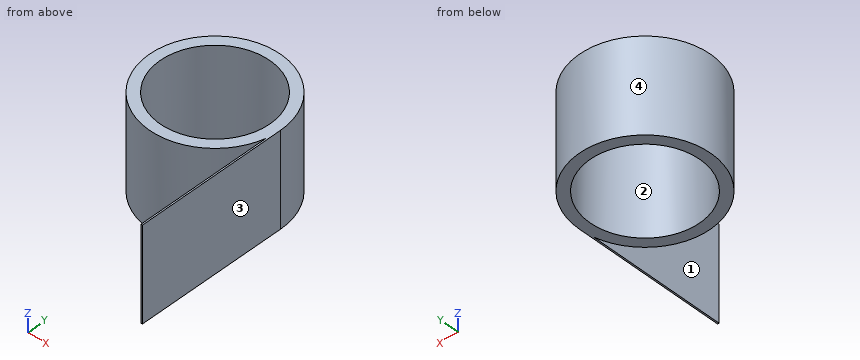
```python
from build123d import *

# Parameters (mm, degrees)
SKETCH1_R           = 11.0871
SKETCH1_R_2         = 9.271
BOSS_EXTRUDE1_DEPTH = 15.875
BOSS_EXTRUDE2_START = -15.875
BOSS_EXTRUDE2_DEPTH = 15.875


with BuildPart() as part:
    # Sketch1 → Boss-Extrude1 (new body)
    with BuildSketch(Plane.XY):
        Circle(SKETCH1_R)
        Circle(SKETCH1_R_2, mode=Mode.SUBTRACT)
    extrude(amount=BOSS_EXTRUDE1_DEPTH)

    # Sketch2 → Boss-Extrude2 (add)
    with BuildSketch(Plane.XY.offset(15.875).offset(BOSS_EXTRUDE2_START)):
        with BuildLine():
            Line((11.0871, 0), (11.0871, -25.4))
            Line((11.0871, -25.4), (10.8331, -25.4))
            Line((10.8331, -25.4), (10.8331, -2.35960395))
            ThreePointArc((10.8331, -2.35960395), (11.023417107, -1.186617756), (11.0871, 0))
        make_face()
    extrude(amount=BOSS_EXTRUDE2_DEPTH)


solid = part.part
```
The model under review builds one solid part; all positions refer to its coordinate system, in mm. Face numbers are marked on the shaded views. A direction names the side the tool comes from. Round coordinates to 2 decimals unless told otherwise and drop trailing zeros. Loops run counter-clockwise (first coordinate to the right, second up) from the corner with the lowest first, then second, coordinate; pieces in that order, holes last. Notation, with made-up numbers: M 80.25,-31.5 L 97.25,-31.5 A15 cw 97.25,-5.5 Z; hole C 58.25,87 d6. An arc over 180 degrees is marked long. Write item = value, one per line.
Item 1: Take a section at B-B on y = -6.5. Write out the cut boundary in (x, z) (3 decimals).
Return value:
outline = M -8.982,0 L -6.611,0 L -6.611,15.875 L -8.982,15.875 Z; M 6.611,0 L 8.982,0 L 8.982,15.875 L 6.611,15.875 Z; M 10.833,0 L 11.087,0 L 11.087,15.875 L 10.833,15.875 Z
Item 2: Take a section at C-C on z = 4.5. Write out the cut boundary in (x, y).
Return value:
outline = M 10.83,-25.4 L 11.09,-25.4 L 11.09,0 A11.09 ccw long 10.83,-2.36 Z; hole C 0,0 d18.54
Item 3: Take a section at A-A on x = 0. Write out the cut boundary in (y, z) (3 decimals), then the cut area to 3 significant figures.
Return value:
outline = M -11.087,0 L -9.271,0 L -9.271,15.875 L -11.087,15.875 Z; M 9.271,0 L 11.087,0 L 11.087,15.875 L 9.271,15.875 Z
area = 57.7 mm2
Item 4: For line 1 (Y direction, x = 0, z = 4); line 2 (X direction, y = -5, z = 3.5); line 3 (X direction, y = -4.5, z = 3.25), list the stretches that pass through material, from the lowest coordinate up. Write a range as [from, to].
Return value:
line_1 = [-11.09, -9.27], [9.27, 11.09]
line_2 = [-9.9, -7.81], [7.81, 9.9], [10.83, 11.09]
line_3 = [-10.13, -8.11], [8.11, 10.13], [10.83, 11.09]
Item 5: Take a section at D-D on y = 4.5. Write out the cut boundary in (x, z) (3 decimals), then the cut area to 3 significant figures.
Return value:
outline = M -10.133,0 L -8.106,0 L -8.106,15.875 L -10.133,15.875 Z; M 8.106,0 L 10.133,0 L 10.133,15.875 L 8.106,15.875 Z
area = 64.4 mm2
Item 6: Insertion check: P1, Ø8, axis at x = -1, z = 7.5, coming from the -Y side; P2, Ø1, axis at x = -8, z = 6.5, coming from the +Y side; P3, Ø5, axis at x = 3, y = 5.5, coming from the -Z side; P4, Ø12, axis at x = -3.5, y = -2.5, coming from the -Z side. Each pin has a flat end and moves straight along its axis. Give the tip position at first contact, or say it passes through.
Return value:
P1 = -11.09
P2 = 8.17
P3 = through
P4 = 0
Item 7: The part is to be moulded in two halves that separate along X. For the marked faces 3 and 4, say which applies: released by +X, released by -X, zero draft, split by the parting line, or undercut.
Return value:
face_3 = released by +X
face_4 = undercut
Item 8: Machinability: for the marked faces 1 and 2, which of the approach directions +Z, -Z, +X, -X, +Y, -Y give a long, thin tool a straight path to every point of the face, cutting with its end or side? Answer none if there is none.
Return value:
face_1 = +Z, -Z, -Y
face_2 = +Z, -Z
